```python
from build123d import *

# Parameters (mm, degrees)
SKETCH_1_W                  = 50
SKETCH_1_H                  = 86
EXTRUDE_1_DEPTH             = 4
SKETCH_2_W                  = 17.5
SKETCH_2_H                  = 22
CUT_EXTRUDE_1_DEPTH         = 5
CUT_EXTRUDE_2_DEPTH         = 3
SKETCH_4_W                  = 7.5
SKETCH_4_H                  = 3
CUT_EXTRUDE_3_DEPTH         = 7.5
SKETCH_5_W                  = 7.5
SKETCH_5_H                  = 3
CUT_EXTRUDE_4_DEPTH         = 7.5
CUT_EXTRUDE_5_DEPTH         = 3
HOLE_WIZARD_3_6_3_6_1_D     = 3.6
HOLE_WIZARD_3_6_3_6_1_DEPTH = 4
FILLET_1_R                  = 3.5


with BuildPart() as part:
    # 草图1 → 凸台-拉伸1 (new body)
    with BuildSketch(Plane(origin=(0, 0, 0), x_dir=(-1, 0, 0), z_dir=(0, 0, -1))):
        with Locations((-600, 300)):
            Rectangle(SKETCH_1_W, SKETCH_1_H)
    extrude(amount=-EXTRUDE_1_DEPTH)

    # 草图2 → 切除-拉伸1 (cut, through all)
    with BuildSketch(Plane.XY.offset(4)):
        with Locations((609.75, 281)):
            Rectangle(SKETCH_2_W, SKETCH_2_H)
    extrude(amount=-CUT_EXTRUDE_1_DEPTH, mode=Mode.SUBTRACT)

    # 草图3 → 切除-拉伸2 (cut)
    with BuildSketch(Plane.XY.offset(4)):
        Polygon((580.675, 258.098814897), (582.35, 261), (580.675, 263.901185103), (577.325, 263.901185103), (575.65, 261), (577.325, 258.098814897), align=None)
    extrude(amount=-CUT_EXTRUDE_2_DEPTH, mode=Mode.SUBTRACT)

    # 草图4 → 切除-拉伸3 (cut)
    with BuildSketch(Plane(origin=(0, 343, 0), x_dir=(-1, 0, 0), z_dir=(0, 1, 0))):
        with Locations((-578.75, 2.5)):
            Rectangle(SKETCH_4_W, SKETCH_4_H)
    extrude(amount=-CUT_EXTRUDE_3_DEPTH, mode=Mode.SUBTRACT)

    # 草图5 → 切除-拉伸4 (cut)
    with BuildSketch(Plane(origin=(0, 343, 0), x_dir=(-1, 0, 0), z_dir=(0, 1, 0))):
        with Locations((-621.25, 2.5)):
            Rectangle(SKETCH_5_W, SKETCH_5_H)
    extrude(amount=-CUT_EXTRUDE_4_DEPTH, mode=Mode.SUBTRACT)

    # 草图6 → 切除-拉伸5 (cut)
    with BuildSketch(Plane.XY.offset(4)):
        Polygon((624.35, 261), (622.675, 263.901185103), (619.325, 263.901185103), (617.65, 261), (619.325, 258.098814897), (622.675, 258.098814897), align=None)
    extrude(amount=-CUT_EXTRUDE_5_DEPTH, mode=Mode.SUBTRACT)

    # Ø3.6 (3.6) 直径孔1
    with Locations(Plane(origin=(0, 0, 0), x_dir=(-1, 0, 0), z_dir=(0, 0, -1))):
        with Locations((-579, 339), (-621, 339), (-579, 261), (-621, 261)):
            Hole(HOLE_WIZARD_3_6_3_6_1_D / 2, depth=HOLE_WIZARD_3_6_3_6_1_DEPTH)

    # 圆角1
    fillet_1_edges = [part.edges().sort_by_distance(p)[0] for p in [
        (582.5, 335.5, 2.5),
        (617.5, 335.5, 2.5),
    ]]
    fillet(fillet_1_edges, radius=FILLET_1_R)


solid = part.part
```
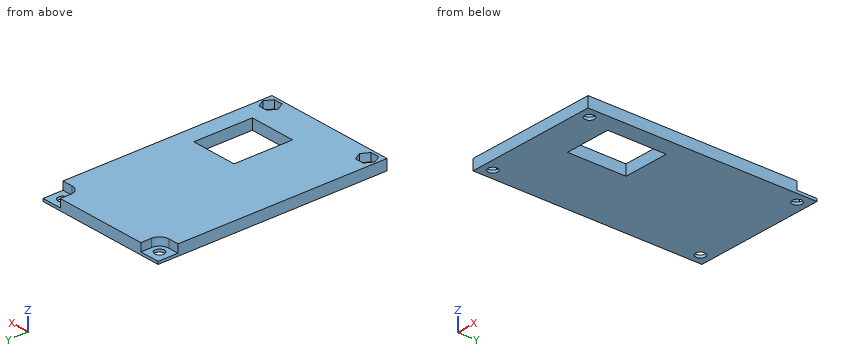
Could you check a few things on this model? Use its own coordinates, in mm. Coordinates: 2 decimals unless noted, no trailing zeros. Loops run counter-clockwise (first coordinate to the right, second up) from the corner with the lowest first, then second, coordinate; pieces in that order, holes last. Notation, with made-up numbers: M -8,11.5 L 2,11.5 A29 cw 2,49.5 Z; hole C 70,-1.75 d2. An arc over 180 degrees is marked long. Put each result on its own line as item: value. Start each with the question number.
(1) Suppose I cut it at B-B on z = 1.85. Please give me the cut outline in (x, y) (3 decimals).
(2) I need wall thicknesses on line 1 (X direction, y = 339, z = 0.5); line 2 (Y direction, x = 579, z = 0.6); line 3 (X direction, y = 288.5, z = 1.9). Which ranges of each line are inside material? Lowest first, please. Write a range as from..to.
(3) Will these pins go through, and if not, where does the flat tip stop? P1, Ø4, axis at x = 621, y = 261, coming from the +Z side; P2, Ø1.5, axis at y = 340.5, z = 2, coming from the -X side.
(4) Suppose I cut it at A-A on y = 290. Please give me the cut outline in (x, z).
Solutions:
1. outline: M 575,257 L 625,257 L 625,335.5 L 621,335.5 A3.5 cw 617.5,339 L 617.5,343 L 582.5,343 L 582.5,339 A3.5 cw 579,335.5 L 575,335.5 Z; hole M 575.65,261 L 577.325,258.099 L 580.675,258.099 L 582.35,261 L 580.675,263.901 L 577.325,263.901 Z; hole M 601,270 L 618.5,270 L 618.5,292 L 601,292 Z; hole M 617.65,261 L 619.325,258.099 L 622.675,258.099 L 624.35,261 L 622.675,263.901 L 619.325,263.901 Z
2. line 1: x = 575..577.2, 580.8..619.2, 622.8..625
2. line 2: y = 257..259.2, 262.8..337.2, 340.8..343
2. line 3: x = 575..601, 618.5..625
3. P1: stops at z = 1
3. P2: stops at x = 582.5
4. outline: M 575,0 L 601,0 L 601,4 L 575,4 Z; M 618.5,0 L 625,0 L 625,4 L 618.5,4 Z
